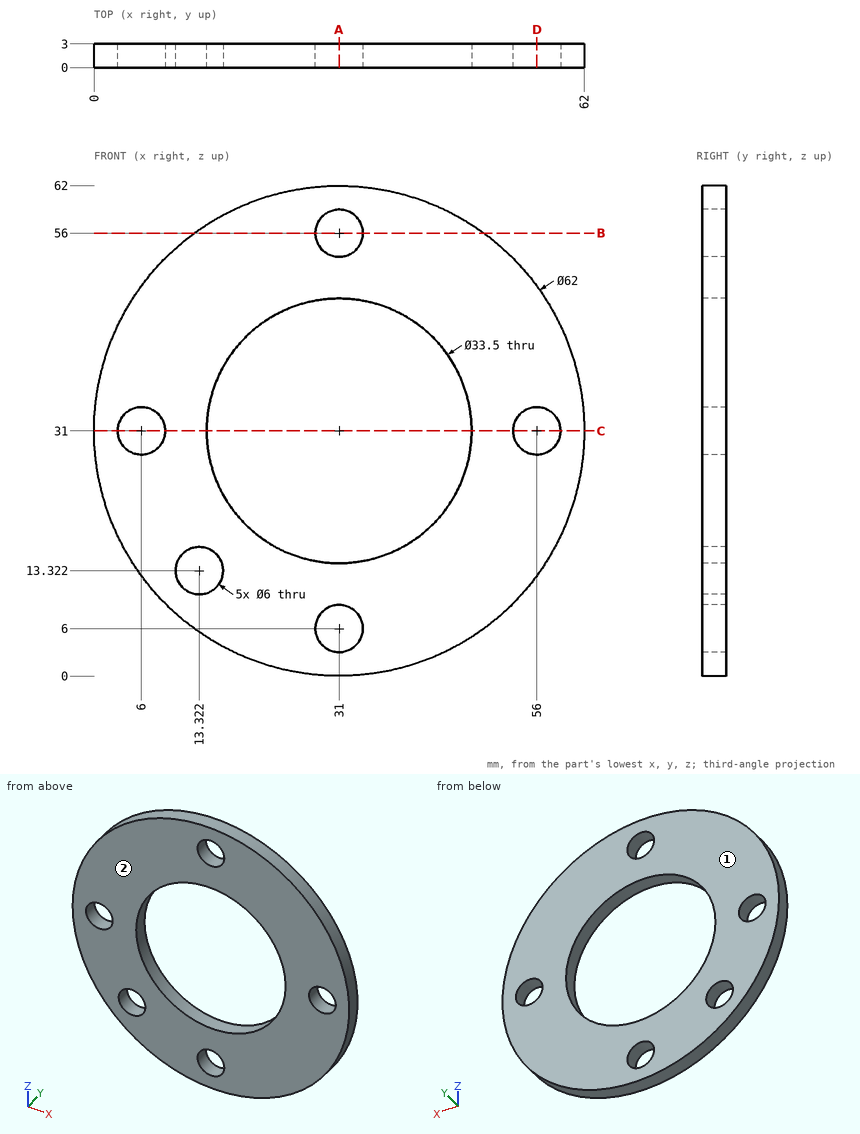
Verification items for this drawing (mm, ordinates from the low corner). Coordinates: 2 decimals unless noted, no trailing zeros. Loops run counter-clockwise (first coordinate to the right, second up) from the corner with the lowest first, then second, coordinate; pieces in that order, holes last.
Item 1: Sectioned sample at C-C, the plane z = 31. Record the boundary of the cut face in (x, y).
Item 2: Sectioned sample at A-A, the plane x = 31. Record the boundary of the cut face in (y, z).
Item 3: Go/stop test with flat-tipped pins: pin 1 Ø20 at (x, z) = (31, 31) entering from +Y; pin 2 Ø1.5 at (x, y) = (29.5, 1.5) entering from -Z. Record where each tip stops, or that it passes through.
Item 4: Release check for a two-part mould opening along Y. For the marked faces 1 and 2 record: released by +Y, released by -Y, zero draft, split by the parting line, or undercut.
Item 5: Sectioned sample at D-D, the plane x = 56. Record the boundary of the cut face in (y, z).
Item 6: Thickness scan on line 1 (Z direction, x = 31, y = 2.3); line 2 (Z direction, x = 29, y = 2.05) (1 decimal); line 3 (Z direction, x = 6, y = 2.1). Record the ranges inside material, lowest first.
Item 7: Sectioned sample at B-B, the plane z = 56. Record the boundary of the cut face in (x, y).
Check result:
1. outline: (0, 0) - (3, 0) - (3, 3) - (0, 3) - close; (9, 0) - (14.25, 0) - (14.25, 3) - (9, 3) - close; (47.75, 0) - (53, 0) - (53, 3) - (47.75, 3) - close; (59, 0) - (62, 0) - (62, 3) - (59, 3) - close
2. outline: (0, 0) - (3, 0) - (3, 3) - (0, 3) - close; (0, 9) - (3, 9) - (3, 14.25) - (0, 14.25) - close; (0, 47.75) - (3, 47.75) - (3, 53) - (0, 53) - close; (0, 59) - (3, 59) - (3, 62) - (0, 62) - close
3. pin 1: passes through
3. pin 2: stops at z = 0.01
4. face 1: released by +Y
4. face 2: released by -Y
5. outline: (0, 12.67) - (3, 12.67) - (3, 28) - (0, 28) - close; (0, 34) - (3, 34) - (3, 49.33) - (0, 49.33) - close
6. line 1: z = 0 to 3, 9 to 14.25, 47.75 to 53, 59 to 62
6. line 2: z = 0.1 to 3.8, 8.2 to 14.4, 47.6 to 53.8, 58.2 to 61.9
6. line 3: z = 12.67 to 28, 34 to 49.33
7. outline: (12.67, 0) - (28, 0) - (28, 3) - (12.67, 3) - close; (34, 0) - (49.33, 0) - (49.33, 3) - (34, 3) - close
